CAD build for the part. Positions are in the model's coordinates, mm. Round coordinates to 2 decimals unless told otherwise and drop trailing zeros. Write each loop counter-clockwise with the first axis right and the second up, starting at its lowest first coordinate (ties: lowest second). Pieces come first, ordered by that corner, then holes. Notation, with made-up numbers: (-6.5, 53) - (38.5, 53) arc R26 ccw to (38.5, 77) - close; hole circle Ø10 at (29.5, 36.5). An arc over 180 degrees is marked (long way). Answer in a Markdown table with one row per item.
Autodesk Inventor part; units mm, degrees
ref_plane "YZ Plane" through (0, 0, 0) normal (1, 0, 0) x (0, 1, 0)
ref_plane "XZ Plane" through (0, 0, 0) normal (0, 1, 0) x (-1, 0, 0)
ref_plane "XY Plane" through (0, 0, 0) normal (0, 0, 1) x (1, 0, 0)
sketch "Sketch1" plane through (0, 0, 0) normal (0, 1, 0) x (-1, 0, 0)
  line L0 (0, 0) -> (168.275, 0)
  line L1 (168.275, 0) -> (168.275, -241.3)
  line L2 (168.275, -241.3) -> (0, -241.3)
  line L3 (0, -241.3) -> (0, 0)
  dimension "d0" = 168.275
  dimension "d1" = 241.3
extrude "Extrusion1" add sketch "Sketch1" along normal blind 19.05
sketch "Sketch2" plane through (0, 19.05, 0) normal (0, 1, 0) x (1, 0, 0)
  circle A0 centre (-63.5, 38.1) radius 14.986
  circle A1 centre (-71.501, 101.092) radius 14.986
  circle A2 centre (-85.471, 133.858) radius 14.986
  circle A3 centre (-99.441, 166.624) radius 14.986
  circle A4 centre (-99.441, 202.6158) radius 14.986
  circle A5 centre (-35.56, 101.092) radius 14.986
  circle A6 centre (-49.53, 133.858) radius 14.986
  circle A7 centre (-63.5, 166.624) radius 14.986
  circle A8 centre (-63.5, 202.6158) radius 14.986
  line L0 (0, 0) -> (-168.275, 0)
  circle A9 centre (-120.65, 82.55) radius 11.7475
  circle A10 centre (-120.65, 114.3) radius 11.7475
  line L1 (0, 0) -> (0, 241.3)
  dimension "d4" = 29.972
  dimension "d5" = 29.972
  dimension "d6" = 29.972
  dimension "d7" = 29.972
  dimension "d8" = 29.972
  dimension "d9" = 29.972
  dimension "d10" = 29.972
  dimension "d11" = 29.972
  dimension "d12" = 29.972
  dimension "d13" = 62.992
  dimension "d14" = 62.992
  dimension "d15" = 32.766
  dimension "d16" = 32.766
  dimension "d17" = 32.766
  dimension "d18" = 32.766
  dimension "d19" = 35.9918
  dimension "d20" = 35.9918
  dimension "d22" = 13.97
  dimension "d23" = 13.97
  dimension "d24" = 8.001
  dimension "d25" = 8.001
  dimension "d26" = 13.97
  dimension "d27" = 13.97
  dimension "d28" = 13.97
  dimension "d29" = 38.1
  dimension "d30" = 23.495
  dimension "d31" = 82.55
  dimension "d33" = 23.495
  dimension "d35" = 31.75
  dimension "d38" = 63.5
  dimension "d39" = 8.001
  dimension "d40" = 120.65
  dimension "d41" = 120.65
extrude "Extrusion2" cut sketch "Sketch2" against normal blind 25.4
properties part number "controlBoard"
Q1. Pull direction X, two halves, no side cores. Call faces 1 (the flat face through (-85, 9, -241.3)), 2 (the flat face through (0, 9, -122)), 3 (the flat face through (-168.275, 9, -119)), 4 (the cylindrical face through (-109.8, 9.7, -109.8)): released by +X, released by -X, zero draft, split by the parting line, or undercut.
Computed:
| item | result |
|---|---|
| face 1 | zero draft |
| face 2 | released by +X |
| face 3 | released by -X |
| face 4 | undercut |
Q2. Saw through at C-C on y = 15.75. Count the separate pieces of the cut face and the enclosed holes in it, then the cut area to 3 significant figures.
Computed:
| item | result |
|---|---|
| separate pieces | 1 |
| enclosed holes | 11 |
| area | 33,400 mm2 |
Q3. Drill centre lines: line 1 (Z direction, x = -120.65, y = 13.25); line 2 (X direction, y = 2.5, z = -134) (3 decimals); line 3 (Z direction, x = -118, y = 4.5). Where is each one in solid material? Low to high.
Computed:
| item | result |
|---|---|
| line 1 | z = -241.3 to -126.05, -102.55 to -94.3, -70.8 to 0 |
| line 2 | x = -168.275 to -100.456, -70.486 to -64.515, -34.545 to 0 |
| line 3 | z = -241.3 to -125.74, -102.86 to -93.99, -71.11 to 0 |
Q4. Saw through at B-B on z = -38.1. List the corners of the cut face in (x, y) (3 decimals).
Computed:
| item | result |
|---|---|
| outline | (-168.275, 0) - (-78.486, 0) - (-78.486, 19.05) - (-168.275, 19.05) - close; (-48.514, 0) - (0, 0) - (0, 19.05) - (-48.514, 19.05) - close |
Q5. Saw through at A-A on x = -120.65. List the corners of the cut face in (y, z).
Computed:
| item | result |
|---|---|
| outline | (0, -241.3) - (19.05, -241.3) - (19.05, -126.05) - (0, -126.05) - close; (0, -102.55) - (19.05, -102.55) - (19.05, -94.3) - (0, -94.3) - close; (0, -70.8) - (19.05, -70.8) - (19.05, 0) - (0, 0) - close |
